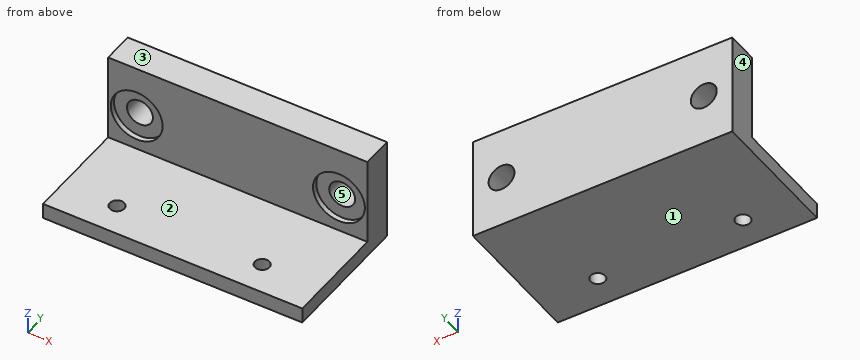
Autodesk Fusion 360 part; units mm, degrees
sketch "Sketch1" plane through (0, 0, 0) normal (0, 0, 1) x (1, 0, 0)
  line L0 (25, -10) -> (-25, -10)
  line L1 (-25, -10) -> (-25, 10)
  line L2 (-25, 10) -> (25, 10)
  line L3 (25, 10) -> (25, -10)
  line L4 (25, -10) -> (-25, 10) construction
  line L5 (-25, -10) -> (25, 10) construction
  line L6 (25, 10) -> (-25, 10)
  line L7 (-25, 10) -> (-25, 16)
  line L8 (-25, 16) -> (25, 16)
  line L9 (25, 16) -> (25, 10)
  dimension "d1" = 50
  dimension "d2" = 20
  dimension "d3" = 6
  dimension "d27" = 50
extrude "Extrude1" add sketch "Sketch1" along normal blind 3 contours L0 L1 L2 L3 L6
extrude "Extrude2" add sketch "Sketch1" along normal blind 20 contours L2 L6 L7 L8 L9
sketch "Sketch2" plane through (0, 16, 0) normal (0, 1, 0) x (-1, 0, 0)
  line L0 (-25, 0) -> (25, 0)
  line L1 (25, 0) -> (25, 20)
  line L2 (25, 20) -> (-25, 20)
  line L3 (-25, 20) -> (-25, 0)
  circle A0 centre (19.5, 10) radius 2.5
  circle A1 centre (-19.5, 10) radius 2.5
  circle A2 centre (-19.5, 10) radius 5
  circle A3 centre (19.5, 10) radius 5
  dimension "d8" = 5
  dimension "d9" = 5
  dimension "d10" = 5.5
  dimension "d11" = 5.5
  dimension "d12" = 10
  dimension "d13" = 10
extrude "Extrude3" cut sketch "Sketch2" against normal up to surface (6 mm away) contours A0 | A1
extrude "Extrude4" cut sketch "Sketch2" along normal blind 1 from surface at -6 contours A2 | A3
sketch "Sketch3" plane through (0, 0, 0) normal (0, 0, -1) x (1, 0, 0)
  line L0 (25, -16) -> (25, 10)
  line L1 (25, 10) -> (-25, 10)
  line L2 (-25, 10) -> (-25, -16)
  line L3 (-25, -16) -> (25, -16)
  circle A0 centre (-14.5, 4) radius 1.4
  circle A1 centre (13.5, 4) radius 1.4
  dimension "d19" = 2.8
  dimension "d20" = 2.8
  dimension "d21" = 28
  dimension "d22" = 6
  dimension "d23" = 6
  dimension "d24" = 10.5
extrude "Extrude5" cut sketch "Sketch3" against normal up to surface (3 mm away) contours A0 | A1
equation "d11 = d10"
equation "d23 = d22"
equation "d24 = ( 50 mm - 29 mm ) / 2"
equation "d27 = d1"
Check sheet for the modelled part. Datum: model origin and axes. Units: mm. Face numbers are marked on the shaded views. A direction names the side the tool comes from. Round coordinates to 2 decimals unless told otherwise and drop trailing zeros. Write each loop counter-clockwise with the first axis right and the second up, starting at its lowest first coordinate (ties: lowest second). Pieces come first, ordered by that corner, then holes. Notation, with made-up numbers: M 65,46.5 L 95,46.5 A12 cw 95,66.5 Z; hole C 41,39 d5. An arc over 180 degrees is marked long. Write item = value, one per line. Start each with the question number.
1. Scan lines: line 1 (Z direction, x = -19.5, y = 10.4); line 2 (X direction, y = 14.75, z = 8.5); line 3 (X direction, y = 12, z = 11.75). Record each from-to range of solid material in increasing order. Write a range as [from, to].
2. Gauge pin test, flat ends, axial feed: pin 1 (6 mm diameter, centred on y = -4.5, z = 4.5, fed in from +X); pin 2 (5 mm diameter, centred on x = -18, z = 11, fed in from -Y); pin 3 (4 mm diameter, centred on x = -17, y = -4.5, fed in from +Z); pin 4 (8 mm diameter, centred on x = 18.5, z = 9.5, fed in from -Y). Record the tip position at first contact, or that the pin passes through.
3. Section check A-A, the plane y = -4. Record the cut outline in (x, z).
4. Section check C-C, the plane z = 10. Record the cut outline in (x, y), then the cut area to 3 significant figures.
5. Section check B-B, the plane x = -19.5. Record the cut outline in (y, z), then the cut area to 3 significant figures.
6. Release check for a two-part mould opening along X. For the marked faces 3, 4 and 5 record: pulls with the +X half, pulls with the -X half, needs draft (parallel to the pull), parting line crosses it, or undercut.
7. Tool access check on the marked faces 1 and 2. Record the directions out of +Z, -Z, +X, -X, +Y, -Y that give a thin tool (end or side, any length) a straight path to the whole face; none if there is none.
8. Section check D-D, the plane x = 13.5. Record the cut outline in (y, z), then the cut area to 3 significant figures.
Results found:
q1.line_1 = [0, 5], [15, 20]
q1.line_2 = [-25, -21.5], [-17.5, 17.5], [21.5, 25]
q1.line_3 = [-25, -21.29], [-17.71, 17.71], [21.29, 25]
q2.pin_1 = 25
q2.pin_2 = 11
q2.pin_3 = 3
q2.pin_4 = 10
q3.outline = M -25,0 L -15.9,0 L -15.9,3 L -25,3 Z; M -13.1,0 L 12.1,0 L 12.1,3 L -13.1,3 Z; M 14.9,0 L 25,0 L 25,3 L 14.9,3 Z
q4.outline = M -25,10 L -24.5,10 L -24.5,11 L -22,11 L -22,16 L -25,16 Z; M -17,11 L -14.5,11 L -14.5,10 L 14.5,10 L 14.5,11 L 17,11 L 17,16 L -17,16 Z; M 22,11 L 24.5,11 L 24.5,10 L 25,10 L 25,16 L 22,16 Z
q4.area = 230 mm^2
q5.outline = M -10,0 L 16,0 L 16,7.5 L 11,7.5 L 11,5 L 10,5 L 10,3 L -10,3 Z; M 10,15 L 11,15 L 11,12.5 L 16,12.5 L 16,20 L 10,20 Z
q5.area = 145 mm^2
q6.face_3 = needs draft
q6.face_4 = pulls with the -X half
q6.face_5 = undercut
q7.face_1 = -Z, +X, -X, +Y, -Y
q7.face_2 = +Z, +X, -X, -Y
q8.outline = M -10,0 L -5.4,0 L -5.4,3 L -10,3 Z; M -2.6,0 L 16,0 L 16,20 L 10,20 L 10,3 L -2.6,3 Z
q8.area = 172 mm^2
